Read the model definition and answer for the solid it produces. Units are mm, in the model's axes. A direction names the side the tool comes from. Round coordinates to 2 decimals unless told otherwise and drop trailing zeros. Loops run counter-clockwise (first coordinate to the right, second up) from the corner with the lowest first, then second, coordinate; pieces in that order, holes last. Notation, with made-up numbers: (17, 32) - (48, 32) arc R34 cw to (48, 71) - close; hole circle Ø8 at (-14, 84.25). An arc over 180 degrees is marked (long way). Answer as CSV lines item,"result".
```python
from build123d import *

# Parameters (mm, degrees)
SKETCH1_R           = 20
BOSS_EXTRUDE1_DEPTH = 110
SKETCH2_R           = 3
CUT_EXTRUDE1_DEPTH  = 25
SKETCH3_R           = 4.5
BOSS_EXTRUDE2_DEPTH = 30
FILLET1_R           = 10
BOSS_EXTRUDE3_REACH = 52
SKETCH4_R           = 2.5


with BuildPart() as part:
    # Sketch1 → Boss-Extrude1 (new body)
    with BuildSketch(Plane(origin=(0, 0, 0), x_dir=(1, 0, 0), z_dir=(0, 1, 0))):
        Circle(SKETCH1_R)
    extrude(amount=BOSS_EXTRUDE1_DEPTH)

    # Sketch2 → Cut-Extrude1 (cut)
    with BuildSketch(Plane(origin=(0, 0, 0), x_dir=(1, 0, 0), z_dir=(0, 1, 0))):
        with Locations((15, 0)):
            Circle(SKETCH2_R)
        with Locations((-15, 0)):
            Circle(SKETCH2_R)
    extrude(amount=CUT_EXTRUDE1_DEPTH, mode=Mode.SUBTRACT)

    # Sketch3 → Boss-Extrude2 (add)
    with BuildSketch(Plane(origin=(0, 0, 0), x_dir=(1, 0, 0), z_dir=(0, 1, 0))):
        Circle(SKETCH3_R)
    extrude(amount=-BOSS_EXTRUDE2_DEPTH)

    # Fillet1
    fillet1_edges = [part.edges().sort_by_distance(p)[0] for p in [
        (-20, 110, 0),
    ]]
    fillet(fillet1_edges, radius=FILLET1_R)

    # Sketch4 → Boss-Extrude3 (add, up to next)
    with BuildSketch(Plane(origin=(30, 0, 0), x_dir=(0, 0, -1), z_dir=(1, 0, 0)), mode=Mode.PRIVATE) as boss_extrude3_sk1:
        with Locations((5, 90)):
            Circle(SKETCH4_R)
    boss_extrude3_tool1 = extrude(boss_extrude3_sk1.sketch, amount=-BOSS_EXTRUDE3_REACH, mode=Mode.PRIVATE) - part.part
    add(boss_extrude3_tool1.solids().sort_by_distance((30, 90, -5))[0])
    # Sketch4 → Boss-Extrude3 (add, up to next)
    with BuildSketch(Plane(origin=(30, 0, 0), x_dir=(0, 0, -1), z_dir=(1, 0, 0)), mode=Mode.PRIVATE) as boss_extrude3_sk2:
        with Locations((-5, 90)):
            Circle(SKETCH4_R)
    boss_extrude3_tool2 = extrude(boss_extrude3_sk2.sketch, amount=-BOSS_EXTRUDE3_REACH, mode=Mode.PRIVATE) - part.part
    add(boss_extrude3_tool2.solids().sort_by_distance((30, 90, 5))[0])


solid = part.part
```
1) Find the intervals of material crossed by line 1 (X direction, y = 13.75, z = 0); line 2 (Y direction, x = 2, z = -9); line 3 (Z direction, x = 15, y = 14), in increasing order.
Entries:
line 1,"x = -20 to -18, -12 to 12, 18 to 20"
line 2,"y = 0 to 110"
line 3,"z = -13.23 to -3, 3 to 13.23"
2) A cutting plane is placed at A-A, the plane y = 90. Determine the outline of the cut face in (x, z).
Entries:
outline,"(18.54, -7.5) - (30, -7.5) - (30, -2.5) - (19.84, -2.5) arc R20 ccw to (19.84, 2.5) - (30, 2.5) - (30, 7.5) - (18.54, 7.5) arc R20 ccw (long way) to start"
3) The mould has two halves that part along Z. Classify faces 4 (the face through (-0.59, -14.79, -4.46)), 5 (the face through (30, 90, -5)), 6 (the face through (-15, 25, 0)): pulls with the +Z half, pulls with the -Z half, needs draft (parallel to the pull), parting line crosses it, or undercut.
Entries:
face 4,"parting line crosses it"
face 5,"needs draft"
face 6,"undercut"
4) A tool of negligible diameter and unlimited length cuts with its end or side. For faces 1 (the face through (0, -30, 0)), 2 (the face through (24.35, 90.751, -7.385)), 3 (the face through (15, 25, 0)), from which of +Z, -Z, +X, -X, +Y, -Y can it reach the whole face along a straight path? Write none if from no direction.
Entries:
face 1,"+Z, -Z, +X, -X, -Y"
face 2,"+X"
face 3,"-Y"
5) Each of these flat-tipped pins is pushed along its axis until it touches: P1, Ø5.5, axis at x = 15, z = 0, coming from the -Y side; P2, Ø10, axis at y = 84.5, z = -5.5, coming from the -X side; P3, Ø1, axis at x = 16, y = 71.5, coming from the +Z side; P4, Ø12, axis at x = 7, z = -1.5, coming from the -Y side. Where does it stop, or does it pass through?
Entries:
P1,"stops at y = 25"
P2,"stops at x = -19.99"
P3,"stops at z = 12.64"
P4,"stops at y = -30"
6) A cutting plane is placed at B-B, the plane y = -1.5. Determine the outline of the cut face in (x, z).
Entries:
outline,"circle Ø9 at (0, 0)"
